Here's how the part is built. I have some questions about the finished solid (model axes, mm). A direction names the side the tool comes from. Give positions to 0.01 mm unless a question says otherwise; leave off trailing zeros. Write each loop counter-clockwise with the first axis right and the second up, starting at its lowest first coordinate (ties: lowest second). Pieces come first, ordered by that corner, then holes. Notation, with made-up numbers: M 24.25,-11 L 39.25,-11 A13 ccw 39.25,-1 Z; hole C 15,4 d8. An arc over 180 degrees is marked long. Use one line per item in the form item = value. Start each with the question number.
from build123d import *

# Parameters (mm, degrees)
F0_W     = 152.4
F0_H     = 76.2
F1_DEPTH = 19.05
F2_T     = -1.21412
F3_W     = 1.9790156
F3_H     = 1.9790156
F4_DEPTH = 19.051
F5_R     = 0.7648956
F6_R     = 1.9790156


with BuildPart() as f1:
    # F0 (on Top) → F1 (new body)
    with BuildSketch(Plane.XY):
        Rectangle(F0_W, F0_H)
    extrude(amount=F1_DEPTH)

    # F2
    f2_openings = [f1.faces().sort_by_distance(p)[0] for p in [
        (0, 0, 19.05),
    ]]
    offset(amount=F2_T, openings=f2_openings)

    # F3 (on face) → F4 (cut, through all)
    with BuildSketch(Plane.XY.offset(19.05)):
        with Locations((-75.2104922, -37.1104922)):
            Rectangle(F3_W, F3_H)
        with Locations((-75.2104922, 37.1104922)):
            Rectangle(F3_W, F3_H)
        with Locations((75.2104922, -37.1104922)):
            Rectangle(F3_W, F3_H)
        with Locations((75.2104922, 37.1104922)):
            Rectangle(F3_W, F3_H)
    extrude(amount=-F4_DEPTH, mode=Mode.SUBTRACT)

    # F5
    f5_edges = [f1.edges().sort_by_distance(p)[0] for p in [
        (-74.98588, 0, 1.21412),
        (0, 36.88588, 1.21412),
        (0, -36.88588, 1.21412),
        (74.98588, 0, 1.21412),
    ]]
    fillet(f5_edges, radius=F5_R)

    # F6
    f6_edges = [f1.edges().sort_by_distance(p)[0] for p in [
        (0, 38.1, 0),
        (-76.2, 0, 0),
        (76.2, 0, 0),
        (0, -38.1, 0),
    ]]
    fillet(f6_edges, radius=F6_R)


solid = f1.part
1) Suppose I cut it at C-C, the plane x = -46.5. List the corners of the cut face in (y, z) for me.
2) Suppose I cut it at A-A, the plane z = 12.75. List the corners of the cut face in (x, y) for me, and give its area (3 significant figures).
3) On a 3-axis mill with a long thin cutter (end or side, diameter ignored), from which of +Z, -Z, +X, -X, +Y, -Y can I reach the whole of each face in a straight line? I mean faces 1 (the face through (-1, 36.886, 10)), 2 (the face through (-76.2, -1, 10)), 3 (the face through (74.986, -1, 10)). Say none if no direction works.
4) Thinking about a two-plate mould opening in X: for faces 4 (the face through (-1, 1, 1.214)), 5 (the face through (-1, 38.1, 10)), 6 (the face through (-74.986, -1, 10)), 7 (the face through (76.2, -1, 10)), which applies, released by +X, released by -X, zero draft, split by the parting line, or undercut?
5) Please list where these lines run through material, in increasing order: line 1 (X direction, y = -14, z = 2.5); line 2 (Y direction, x = 48, z = 6.75); line 3 (Z direction, x = 52, y = -29.5).
6) Suppose I cut it at B-B, the plane y = -3. List the corners of the cut face in (x, z) for me.
7) Will these pins go through, and if not, where does the flat tip stop? P1, Ø1.6, axis at x = 75.5, z = 14, coming from the +Y side; P2, Ø12, axis at x = -60.5, y = 24, coming from the +Z side; P3, Ø1.6, axis at y = -37.5, z = 10.5, coming from the -X side.
Checks:
q1.outline = M -38.1,1.98 A1.98 ccw -36.12,0 L 36.12,0 A1.98 ccw 38.1,1.98 L 38.1,19.05 L 36.89,19.05 L 36.89,1.98 A0.76 cw 36.12,1.21 L -36.12,1.21 A0.76 cw -36.89,1.98 L -36.89,19.05 L -38.1,19.05 Z
q2.outline = M -76.2,-36.12 L -74.99,-36.12 L -74.99,36.12 L -76.2,36.12 Z; M -74.22,-38.1 L 74.22,-38.1 L 74.22,-36.89 L -74.22,-36.89 Z; M -74.22,36.89 L 74.22,36.89 L 74.22,38.1 L -74.22,38.1 Z; M 74.99,-36.12 L 76.2,-36.12 L 76.2,36.12 L 74.99,36.12 Z
q2.area = 536 mm^2
q3.face_1 = +Z, +X, -X
q3.face_2 = +Z, -Z, -X, +Y, -Y
q3.face_3 = +Z, +Y, -Y
q4.face_4 = undercut
q4.face_5 = zero draft
q4.face_6 = undercut
q4.face_7 = released by +X
q5.line_1 = -76.2 to -74.99, 74.99 to 76.2
q5.line_2 = -38.1 to -36.89, 36.89 to 38.1
q5.line_3 = 0 to 1.21
q6.outline = M -76.2,1.98 A1.98 ccw -74.22,0 L 74.22,0 A1.98 ccw 76.2,1.98 L 76.2,19.05 L 74.99,19.05 L 74.99,1.98 A0.76 cw 74.22,1.21 L -74.22,1.21 A0.76 cw -74.99,1.98 L -74.99,19.05 L -76.2,19.05 Z
q7.P1 = 36.12
q7.P2 = 1.21
q7.P3 = -74.22
